Geometry check sheet. Reference: the model listing, model coordinates, mm. A direction names the side the tool comes from. Coordinates: 2 decimals unless noted, no trailing zeros. Loops run counter-clockwise (first coordinate to the right, second up) from the corner with the lowest first, then second, coordinate; pieces in that order, holes last.
from build123d import *

# Parameters (mm, degrees)
SKIZZE1_W                       = 24
SKIZZE1_H                       = 16
AUFSATZ_LINEAR_AUSTRAGEN1_DEPTH = 3
AUFSATZ_LINEAR_AUSTRAGEN2_DEPTH = 10.8


with BuildPart() as part:
    # Skizze1 → Aufsatz-Linear austragen1 (new body)
    with BuildSketch(Plane.XY):
        Rectangle(SKIZZE1_W, SKIZZE1_H)
    extrude(amount=AUFSATZ_LINEAR_AUSTRAGEN1_DEPTH)

    # Skizze2 → Aufsatz-Linear austragen2 (add)
    with BuildSketch(Plane.XY.offset(3)):
        with BuildLine():
            ThreePointArc((-3.999695252, 7.950625), (-6.26249607, 6.323855072), (-7.911250653, 4.077022578))
            ThreePointArc((-7.911250653, 4.077022578), (-3.876728126, 0.037983649), (-7.989616413, -3.92122807))
            ThreePointArc((-7.989616413, -3.92122807), (-6.304514257, -6.281966252), (-3.949828748, -7.975515837))
            ThreePointArc((-3.949828748, -7.975515837), (0.022550329, -3.799433377), (4.044219423, -7.928069706))
            ThreePointArc((4.044219423, -7.928069706), (6.359488738, -6.226307332), (8.011875714, -3.875544807))
            ThreePointArc((8.011875714, -3.875544807), (3.923312373, 0.061138188), (7.88722716, 4.123305437))
            ThreePointArc((7.88722716, 4.123305437), (6.243943055, 6.342174322), (3.999695252, 7.950625))
            ThreePointArc((3.999695252, 7.950625), (0, 4), (-3.999695252, 7.950625))
        make_face()
    extrude(amount=AUFSATZ_LINEAR_AUSTRAGEN2_DEPTH)

    # Skizze3 → Schnitt-Rotation1 (revolve, cut)
    with BuildSketch(Plane(origin=(0, 0, 0), x_dir=(1, 0, 0), z_dir=(0, 1, 0))):
        with BuildLine():
            Line((0, -4), (0, -16))
            ThreePointArc((0, -16), (6, -10), (0, -4))
        make_face()
    revolve(axis=Axis((0, 0, 4), (0, 0, 1)), mode=Mode.SUBTRACT)


solid = part.part
1) Material ranges on probe 1 along Z at (x, y) = (-4.25, -0.75); probe 2 along Y at (x, z) = (5.75, 3.75); probe 3 along X at (y, z) = (3.25, 6.25), recorded low to high.
Data:
probe 1: z = 0 to 3
probe 2: y = -6.79 to -3.23, 3.48 to 6.79
probe 3: x = -5.44 to -3.37, 3.37 to 5.43
2) Section check A-A on y = -2.5. Record the cut outline in (x, z).
Data:
outline: (-12, 0) - (12, 0) - (12, 3) - (4.9, 3) - (4.9, 7.61) arc R5.45 cw to (-4.82, 7.44) - (-4.82, 3) - (-12, 3) - close; (-4.82, 12.56) arc R5.45 cw to (-3.91, 13.8) - (-4.82, 13.8) - close; (3.91, 13.8) arc R5.45 cw to (4.9, 12.39) - (4.9, 13.8) - close
3) Section check B-B on z = 12.5. Record the cut outline in (x, y), and give its area (3 significant figures).
Data:
outline: (-7.99, -3.92) arc R8.9 ccw to (-3.95, -7.98) arc R4 cw to (-2.6, -4.8) arc R5.45 cw to (-4.84, -2.52) arc R4 cw to start; (-7.91, 4.08) arc R4 cw to (-4.79, 2.62) arc R5.45 cw to (-2.48, 4.86) arc R4 cw to (-4, 7.95) arc R8.9 ccw to start; (2.48, 4.86) arc R5.45 cw to (4.79, 2.61) arc R4 cw to (7.89, 4.12) arc R8.9 ccw to (4, 7.95) arc R4 cw to start; (2.65, -4.77) arc R4 cw to (4.04, -7.93) arc R8.9 ccw to (8.01, -3.88) arc R4 cw to (4.87, -2.46) arc R5.45 cw to start
area: 54.4 mm2
4) Section check C-C on x = 2.75. Record the cut outline in (y, z).
Data:
outline: (-8, 0) - (8, 0) - (8, 3) - (5.1, 3) - (5.1, 8.43) arc R5.33 cw to (-4.85, 7.79) - (-4.85, 3) - (-8, 3) - close; (-4.85, 12.21) arc R5.33 cw to (-3.74, 13.8) - (-4.85, 13.8) - close; (3.74, 13.8) arc R5.33 cw to (5.1, 11.57) - (5.1, 13.8) - close
5) Section check D-D on x = -6. Record the cut outline in (y, z).
Data:
outline: (-8, 0) - (8, 0) - (8, 3) - (6.57, 3) - (6.57, 13.8) - (3.61, 13.8) - (3.61, 3) - (-3.46, 3) - (-3.46, 13.8) - (-6.57, 13.8) - (-6.57, 3) - (-8, 3) - close
6) Access from +Z, -Z, +X, -X, +Y, -Y to the whole of each face (thin tool, end or side, straight path). Record for faces 4 (the cylindrical face through (2.62, 4.98, 7.12)), 5 (the cylindrical face through (6.331, -6.255, 8.324)), 6 (the cylindrical face through (-6.235, 6.351, 8.324)), 7 (the cylindrical face through (6.272, 6.315, 8.324)).
Data:
face 4: +Z, +Y
face 5: +Z, +X, -Y
face 6: +Z, -X, +Y
face 7: +Z, +X, +Y
7) Depth check by flat-ended pin: pin 1 (4 mm diameter, centred on y = 1, z = 8.5, fed in from +X); pin 2 (3 mm diameter, centred on x = 3, z = 9, fed in from -Y). Enter the tip coordinate at first touch or a pass-through.
Data:
pin 1: stops at x = 5.14
pin 2: stops at y = -7.93
8) Mould release check, pull along X, two halves, no side actions. Record for faces 1 (the cylindrical face through (-2.661, -4.855, 7.124)), 2 (the cylindrical face through (-6.333, -6.253, 8.324)), 3 (the flat face through (0, -8, 1)): +X half, -X half, draft (parallel to the pull), parting line (faces both ways), or undercut.
Data:
face 1: undercut
face 2: -X half
face 3: draft
